from build123d import *

# Parameters (mm, degrees)
CROQUIS1_R              = 30.5
SALIENTE_EXTRUIR1_DEPTH = 2.4
CORTAR_EXTRUIR3_START   = -4
CORTAR_EXTRUIR3_DEPTH   = 4
CORTAR_EXTRUIR6_DEPTH   = 10
CROQUIS10_R             = 2.5
CORTAR_EXTRUIR7_DEPTH   = 10
CORTAR_EXTRUIR8_START   = -3
CORTAR_EXTRUIR8_DEPTH   = 3
SALIENTE_EXTRUIR2_DEPTH = 10
REDONDEO1_R             = 3
REDONDEO2_R             = 1
CORTAR_EXTRUIR9_START   = -3
CORTAR_EXTRUIR9_DEPTH   = 3
CORTAR_EXTRUIR10_START  = -10
CORTAR_EXTRUIR10_DEPTH  = 10
CROQUIS19_R             = 3
SALIENTE_EXTRUIR5_DEPTH = 7
CROQUIS20_R             = 1.5
CORTAR_EXTRUIR12_DEPTH  = 6
REDONDEO3_R             = 1
REDONDEO4_R             = 1
CORTAR_EXTRUIR13_DEPTH  = 3


with BuildPart() as part:
    # Croquis1 → Saliente-Extruir1 (new body)
    with BuildSketch(Plane(origin=(0, 0, 0), x_dir=(1, 0, 0), z_dir=(0, 1, 0))):
        with Locations(Location((0, 0, 0), (0, 0, 270))):
            Circle(CROQUIS1_R)
    extrude(amount=SALIENTE_EXTRUIR1_DEPTH)

    # Croquis5 → Cortar-Extruir3 (cut)
    with BuildSketch(Plane(origin=(0, 2.4, 0), x_dir=(1, 0, 0), z_dir=(0, 1, 0)).offset(CORTAR_EXTRUIR3_START)):
        with BuildLine():
            Line((28.814059068, 5), (30.087372767, 5))
            ThreePointArc((30.087372767, 5), (29.556634924, 7.526973624), (28.814059068, 10))
            Line((28.814059068, 10), (24.814059068, 10))
            Line((24.814059068, 10), (24.814059068, 5))
            Line((24.814059068, 5), (28.814059068, 5))
        make_face()
        with BuildLine():
            Line((30.087372767, -5), (28.814059068, -5))
            Line((28.814059068, -5), (24.814059068, -5))
            Line((24.814059068, -5), (24.814059068, -10))
            Line((24.814059068, -10), (28.814059068, -10))
            ThreePointArc((28.814059068, -10), (29.556634924, -7.526973624), (30.087372767, -5))
        make_face()
        with BuildLine():
            Line((-24.814059068, 5), (-24.814059068, 10))
            Line((-24.814059068, 10), (-28.814059068, 10))
            ThreePointArc((-28.814059068, 10), (-29.556634924, 7.526973624), (-30.087372767, 5))
            Line((-30.087372767, 5), (-28.814059068, 5))
            Line((-28.814059068, 5), (-24.814059068, 5))
        make_face()
        with BuildLine():
            Line((-28.814059068, -10), (-24.814059068, -10))
            Line((-24.814059068, -10), (-24.814059068, -5))
            Line((-24.814059068, -5), (-28.814059068, -5))
            Line((-28.814059068, -5), (-30.087372767, -5))
            ThreePointArc((-30.087372767, -5), (-29.556634924, -7.526973624), (-28.814059068, -10))
        make_face()
    extrude(amount=CORTAR_EXTRUIR3_DEPTH, mode=Mode.SUBTRACT)

    # Croquis9 → Cortar-Extruir6 (cut)
    with BuildSketch(Plane(origin=(0, 2.4, 0), x_dir=(1, 0, 0), z_dir=(0, 1, 0))):
        Polygon((5.673284852, 12.685390231), (8.887222901, 8.855168016), (11.18535623, 10.783530845), (7.971418181, 14.613753061), align=None)
        Polygon((-2.120514915, 21.973679104), (1.093423133, 18.143456889), (3.391556462, 20.071819718), (0.177618414, 23.902041933), align=None)
    extrude(amount=-CORTAR_EXTRUIR6_DEPTH, mode=Mode.SUBTRACT)

    # Croquis10 → Cortar-Extruir7 (cut)
    with BuildSketch(Plane(origin=(0, 2.4, 0), x_dir=(1, 0, 0), z_dir=(0, 1, 0))):
        with Locations(Location((12, 16, 0), (0, 0, 270))):
            Circle(CROQUIS10_R)
        with Locations(Location((-12, -16, 0), (0, 0, 270))):
            Circle(CROQUIS10_R)
    extrude(amount=-CORTAR_EXTRUIR7_DEPTH, mode=Mode.SUBTRACT)

    # Croquis11 → Cortar-Extruir8 (cut)
    with BuildSketch(Plane(origin=(0, 2.4, 0), x_dir=(1, 0, 0), z_dir=(0, 1, 0)).offset(CORTAR_EXTRUIR8_START)):
        with BuildLine():
            ThreePointArc((-28.814059068, -10), (-28.341972277, -11.268655974), (-27.814059068, -12.515115586))
            Line((-27.814059068, -12.515115586), (-27.814059068, -10))
            Line((-27.814059068, -10), (-28.814059068, -10))
        make_face()
        with BuildLine():
            Line((-27.814059068, -5), (-27.814059068, 5))
            Line((-27.814059068, 5), (-30.087372767, 5))
            ThreePointArc((-30.087372767, 5), (-30.5, 0), (-30.087372767, -5))
            Line((-30.087372767, -5), (-27.814059068, -5))
        make_face()
        with BuildLine():
            Line((-27.814059068, 10), (-27.814059068, 12.515115586))
            ThreePointArc((-27.814059068, 12.515115586), (-28.341972277, 11.268655974), (-28.814059068, 10))
            Line((-28.814059068, 10), (-27.814059068, 10))
        make_face()
        with BuildLine():
            Line((28.814059068, -10), (27.814059068, -10))
            Line((27.814059068, -10), (27.814059068, -12.515115586))
            ThreePointArc((27.814059068, -12.515115586), (28.341972277, -11.268655974), (28.814059068, -10))
        make_face()
        with BuildLine():
            Line((30.087372767, 5), (27.814059068, 5))
            Line((27.814059068, 5), (27.814059068, -5))
            Line((27.814059068, -5), (30.087372767, -5))
            ThreePointArc((30.087372767, -5), (30.5, 0), (30.087372767, 5))
        make_face()
        with BuildLine():
            Line((27.814059068, 12.515115586), (27.814059068, 10))
            Line((27.814059068, 10), (28.814059068, 10))
            ThreePointArc((28.814059068, 10), (28.341972277, 11.268655974), (27.814059068, 12.515115586))
        make_face()
    extrude(amount=CORTAR_EXTRUIR8_DEPTH, mode=Mode.SUBTRACT)

    # Croquis13 → Saliente-Extruir2 (add)
    with BuildSketch(Plane.XZ):
        Polygon((-6.816688183, 4.321977983), (-19.672440377, -10.99891088), (-17.374307048, -12.927273709), (-4.518554854, 2.393615154), align=None)
        Polygon((21.527275636, 8.931176939), (23.455638465, 11.229310268), (11.964971818, 20.871124414), (10.036608989, 18.572991084), align=None)
    extrude(amount=SALIENTE_EXTRUIR2_DEPTH)

    # Redondeo1
    redondeo1_edges = [part.edges().sort_by_distance(p)[0] for p in [
        (-5.667621519, -10, 3.357796568),
        (-18.523373712, -10, -11.963092294),
        (22.49145705, -10, 10.080243604),
        (11.000790403, -10, 19.722057749),
    ]]
    fillet(redondeo1_edges, radius=REDONDEO1_R)

    # Redondeo2
    redondeo2_edges = [part.edges().sort_by_distance(p)[0] for p in [
        (-5.667621519, 0, 3.357796568),
        (-13.24456428, 0, -3.338466449),
        (-18.523373712, 0, -11.963092294),
        (22.49145705, 0, 10.080243604),
        (17.710305141, 0, 16.050217341),
        (11.000790403, 0, 19.722057749),
    ]]
    fillet(redondeo2_edges, radius=REDONDEO2_R)

    # Croquis14 → Cortar-Extruir9 (cut)
    with BuildSketch(Plane(origin=(0, 2.4, 0), x_dir=(1, 0, 0), z_dir=(0, 1, 0)).offset(CORTAR_EXTRUIR9_START)):
        with BuildLine():
            Line((-0.28585192, 30.498660441), (27.814059068, 11.545031156))
            Line((27.814059068, 11.545031156), (27.814059068, 12.515115586))
            ThreePointArc((27.814059068, 12.515115586), (16.440879495, 25.689442995), (-0.28585192, 30.498660441))
        make_face()
    extrude(amount=CORTAR_EXTRUIR9_DEPTH, mode=Mode.SUBTRACT)

    # Croquis15 → Cortar-Extruir10 (cut)
    with BuildSketch(Plane(origin=(0, 2.4, 0), x_dir=(1, 0, 0), z_dir=(0, 1, 0)).offset(CORTAR_EXTRUIR10_START)):
        with BuildLine():
            Line((-27.814059068, -12.24829445), (-27.814059068, -12.515115586))
            ThreePointArc((-27.814059068, -12.515115586), (-16.882746118, -25.401237834), (-0.769174213, -30.490299622))
            Line((-0.769174213, -30.490299622), (-27.814059068, -12.24829445))
        make_face()
    extrude(amount=CORTAR_EXTRUIR10_DEPTH, mode=Mode.SUBTRACT)

    # Croquis19 → Saliente-Extruir5 (add)
    with BuildSketch(Plane(origin=(-14.375575006, 0, 21.312666404), x_dir=(0.8290375725550415, 0, 0.5591929034707471), z_dir=(-0.5591929034707471, 0, 0.8290375725550415))):
        with Locations((10.101272087, 2.4)):
            Circle(CROQUIS19_R)
        with Locations((-9.898727913, 2.4)):
            Circle(CROQUIS19_R)
    extrude(amount=-SALIENTE_EXTRUIR5_DEPTH)

    # Croquis20 → Cortar-Extruir12 (cut)
    with BuildSketch(Plane(origin=(-14.375575006, 0, 21.312666404), x_dir=(0.8290375725550415, 0, 0.5591929034707471), z_dir=(-0.5591929034707471, 0, 0.8290375725550415))):
        with Locations((10.101272087, 2.4)):
            Circle(CROQUIS20_R)
        with Locations((-9.898727913, 2.4)):
            Circle(CROQUIS20_R)
    extrude(amount=-CORTAR_EXTRUIR12_DEPTH, mode=Mode.SUBTRACT)

    # Redondeo3
    redondeo3_edges = [part.edges().sort_by_distance(p)[0] for p in [
        (-2.086890591, 5.4, 21.157963063),
        (-18.667642042, 5.4, 9.974104993),
    ]]
    fillet(redondeo3_edges, radius=REDONDEO3_R)

    # Redondeo4
    redondeo4_edges = [part.edges().sort_by_distance(p)[0] for p in [
        (-27.814059068, 1.2, 10),
        (-27.814059068, 1.2, -10),
        (27.814059068, 1.2, 10),
        (27.814059068, 1.2, -10),
    ]]
    fillet(redondeo4_edges, radius=REDONDEO4_R)

    # Croquis21 → Cortar-Extruir13 (cut)
    with BuildSketch(Plane(origin=(0, 2.4, 0), x_dir=(1, 0, 0), z_dir=(0, 1, 0))):
        Polygon((5.673284852, 12.685390231), (7.971418181, 14.613753061), (7.778581899, 14.843566393), (5.480448569, 12.915203564), align=None)
        Polygon((3.391556462, 20.071819718), (1.093423133, 18.143456889), (1.286259416, 17.913643556), (3.584392745, 19.842006385), align=None)
        Polygon((0.177618414, 23.902041933), (-2.120514915, 21.973679104), (-2.313351198, 22.203492437), (-0.015217869, 24.131855266), align=None)
        Polygon((8.887222901, 8.855168016), (11.18535623, 10.783530845), (11.378192513, 10.553717512), (9.080059183, 8.625354683), align=None)
    extrude(amount=-CORTAR_EXTRUIR13_DEPTH, mode=Mode.SUBTRACT)


solid = part.part
Read the model definition and answer for the solid it produces. Units are mm, in the model's axes. A direction names the side the tool comes from. Give positions to 0.01 mm unless a question says otherwise; leave off trailing zeros. Write each loop counter-clockwise with the first axis right and the second up, starting at its lowest first coordinate (ties: lowest second). Pieces come first, ordered by that corner, then holes. Notation, with made-up numbers: M 11,47 L 58,47 A12 ccw 58,63 Z; hole C 62,86.5 d7. An arc over 180 degrees is marked long. One line per item, written item: value. Start each with the question number.
(1) Flat-ended cylindrical pins translate along their axes: pin 1 Ø1 at (x, y) = (-25.5, 1) entering from -Z; pin 2 Ø1 at (x, y) = (12.5, -6) entering from +Z; pin 3 Ø8 at (x, z) = (-8, 6.5) entering from -Y. Find the tip coordinate at first contact, or state that the pin passes through.
(2) Find section D-D (z = -25). Determine the outline of the cut face in (x, y).
(3) Find the intervals of material crossed by line 1 (X direction, y = 1.8, z = 16); line 2 (Y direction, x = -0.5, z = 11); line 3 (X direction, y = 1.15, z = -16), in increasing order.
(4) Find section C-C (z = 7). Determine the outline of the cut face in (x, y).
(5) Determine the mould class of faces 1 (the cylindrical face through (17.812, -0.285, 16.357)), 2 (the cylindrical face through (10.788, -0.285, 19.936)), 3 (the flat face through (-26, 1, 10)) for opening direction X: pulls with the +X half, pulls with the -X half, needs draft (parallel to the pull), parting line crosses it, or undercut.
(6) Find section B-B (z = -16). Determine the outline of the cut face in (x, y).
(7) Find section A-A (y = -2.25). Determine the outline of the cut face in (x, z), plus the area to 3 significant figures.
(8) A tool of negligible diameter and unlimited length cuts with its end or side. For faces 4 (the flat face through (-11.045, -4.93, -5.385)), 5 (the flat face through (26, 1, 5)), 6 (the flat face through (6.646, 1.217, -13.893)), from which of +Z, -Z, +X, -X, +Y, -Y can it reach the whole face along a straight path? Write none if from no direction.
Results below:
1. pin 1: stops at z = -17.47
1. pin 2: stops at z = 20.84
1. pin 3: stops at y = -9.93
2. outline: M -17.47,0 L 7.87,0 L 7.87,2.4 L -17.47,2.4 Z
3. line 1: x = -21.07 to -14.5, -9.5 to 25.97
3. line 2: y = 0 to 2.4
3. line 3: x = -25.97 to 9.5, 14.5 to 21.21
4. outline: M -24.81,0 L 24.81,0 L 24.81,2.4 L -24.81,2.4 Z
5. face 1: pulls with the +X half
5. face 2: undercut
5. face 3: needs draft
6. outline: M -25.97,0 L 9.5,0 L 9.5,2.4 L -25.97,2.4 Z; M 14.5,0 L 21.21,0 L 21.21,2.4 L 14.5,2.4 Z
7. outline: M -19.67,-11 L -17.37,-12.93 L -4.52,2.39 L -6.82,4.32 Z; M 10.04,18.57 L 21.53,8.93 L 23.46,11.23 L 11.96,20.87 Z
7. area: 105 mm^2
8. face 4: -Z, +X, -Y
8. face 5: +X, +Y, -Y
8. face 6: +Y, -Y
